```python
from build123d import *

# Parameters (mm, degrees)
SKETCH1_R           = 3.2639
BOSS_EXTRUDE1_DEPTH = 4.7625
CUT_EXTRUDE4_DEPTH  = 274.082391315


with BuildPart() as part:
    # Sketch1 → Boss-Extrude1 (new body)
    with BuildSketch(Plane.XY):
        with BuildLine():
            Line((-220.98, 0), (-220.98, -3.2004))
            ThreePointArc((-220.98, -3.2004), (-219.127567548, -7.672567548), (-214.6554, -9.525))
            Line((-214.6554, -9.525), (-190.4746, -9.525))
            ThreePointArc((-190.4746, -9.525), (-186.002432452, -7.672567548), (-184.15, -3.2004))
            Line((-184.15, -3.2004), (-184.15, 0))
            ThreePointArc((-184.15, 0), (-170.132415912, 70.47115407), (-130.213713756, 130.213713756))
            Line((-130.213713756, 130.213713756), (-127.950689213, 132.476738298))
            ThreePointArc((-127.950689213, 132.476738298), (-126.098256761, 136.948905846), (-127.950689213, 141.421073395))
            Line((-127.950689213, 141.421073395), (-145.049096868, 158.519481049))
            ThreePointArc((-145.049096868, 158.519481049), (-149.521264416, 160.371913501), (-153.993431964, 158.519481049))
            Line((-153.993431964, 158.519481049), (-156.256456507, 156.256456507))
            ThreePointArc((-156.256456507, 156.256456507), (-204.158899094, 84.565384884), (-220.98, 0))
        make_face()
        with Locations(Location((-212.09, 0, 0), (0, 0, 180))):
            Circle(SKETCH1_R, mode=Mode.SUBTRACT)
        with Locations(Location((-209.478820157, 33.17818569, 0), (0, 0, 180))):
            Circle(SKETCH1_R, mode=Mode.SUBTRACT)
        with Locations(Location((-201.709576541, 65.539414337, 0), (0, 0, 180))):
            Circle(SKETCH1_R, mode=Mode.SUBTRACT)
        with Locations(Location((-188.973573715, 96.28684509, 0), (0, 0, 180))):
            Circle(SKETCH1_R, mode=Mode.SUBTRACT)
        with Locations(Location((-171.584414337, 124.663374159, 0), (0, 0, 180))):
            Circle(SKETCH1_R, mode=Mode.SUBTRACT)
        with Locations(Location((-149.970277222, 149.970277222, 0), (0, 0, 180))):
            Circle(SKETCH1_R, mode=Mode.SUBTRACT)
        with BuildLine():
            ThreePointArc((-190.318686211, 8.309493293), (-174.366836772, 76.723244418), (-134.703841816, 134.703841816))
            ThreePointArc((-134.703841816, 134.703841816), (-134.703841816, 139.193969877), (-139.193969877, 139.193969877))
            ThreePointArc((-139.193969877, 139.193969877), (-180.179064665, 79.280685899), (-196.662642418, 8.586476403))
            ThreePointArc((-196.662642418, 8.586476403), (-193.62915587, 5.276006744), (-190.318686211, 8.309493293))
        make_face(mode=Mode.SUBTRACT)
    extrude(amount=BOSS_EXTRUDE1_DEPTH)

    # Sketch2 → Cut-Extrude4 (cut, through all)
    with BuildSketch(Plane.XY):
        with BuildLine():
            Line((-202.7174, -9.525), (-183.6674, -9.525))
            Line((-183.6674, -9.525), (-183.6674, 9.525))
            ThreePointArc((-183.6674, 9.525), (-189.247015818, -3.945384182), (-202.7174, -9.525))
        make_face()
    extrude(amount=CUT_EXTRUDE4_DEPTH, mode=Mode.SUBTRACT)


solid = part.part
```
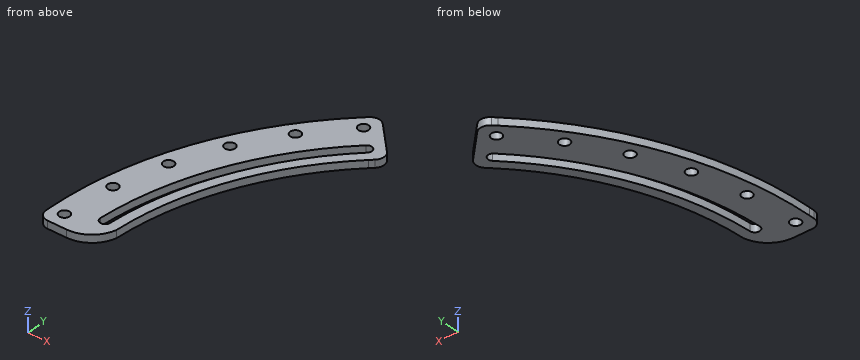
The model under review builds one solid part; all positions refer to its coordinate system, in mm. Coordinates: 2 decimals unless noted, no trailing zeros. Write each loop counter-clockwise with the first axis right and the second up, starting at its lowest first coordinate (ties: lowest second). Pieces come first, ordered by that corner, then holes. Notation, with made-up numbers: (22, 5.25) -> (29, 5.25) arc R27 cw to (29, 32.25) -> close; hole circle Ø1 at (-19, 41.25). An arc over 180 degrees is marked (long way). One line per item, written item: value. Start each with the question number.
Q1. Add section B-B, the plane x = -158.5. Give the boundary of the cut face in (y, z), then the cut area to 3 significant figures.
Q2. Clearance check with flat-ended pins moving along their axes: P1, Ø1.5, axis at x = -142, z = 1.5, coming from the +Y side; P2, Ø1, axis at y = 39, z = 3, coming from the +X side; P3, Ø2, axis at y = 116.5, z = 3.5, coming from the -X side. State where each tip first meets the part, or that it passes through.
Q3. Add section C-C, the plane z = 3.7. Count the separate pieces of the cut face and the enclosed holes in it, then the cut area to 3 significant figures.
Q4. To check wall thickness, follow probe 1 along X at (y, z) = (125, 1.95); probe 2 along X at (y, z) = (32, 4.5); probe 3 along Y at (x, z) = (-150, 2.75). State the ranges of each line that lie inside material, in increasing order.
Q5. Add section A-A, the plane y = 78.5. Give the boundary of the cut face in (x, z), then the cut area to 3 significant figures.
Response:
1. outline: (93.75, 0) -> (105.68, 0) -> (105.68, 4.76) -> (93.75, 4.76) -> close; (116.74, 0) -> (153.98, 0) -> (153.98, 4.76) -> (116.74, 4.76) -> close
1. area: 234 mm²
2. P1: y = 156.22
2. P2: x = -179.86
2. P3: x = -188.39
3. separate pieces: 1
3. enclosed holes: 7
3. area: 5,320 mm²
4. probe 1: -182.23 to -174.83, -168.34 to -152.07, -143.75 to -135.23
4. probe 2: -218.65 to -212.52, -206.43 to -194.23, -187.79 to -181.35
4. probe 3: 106.82 to 117.43, 127.48 to 146.71, 153.23 to 160.35
5. outline: (-206.57, 0) -> (-180.52, 0) -> (-180.52, 4.76) -> (-206.57, 4.76) -> close; (-173.57, 0) -> (-166.58, 0) -> (-166.58, 4.76) -> (-173.57, 4.76) -> close
5. area: 157 mm²
